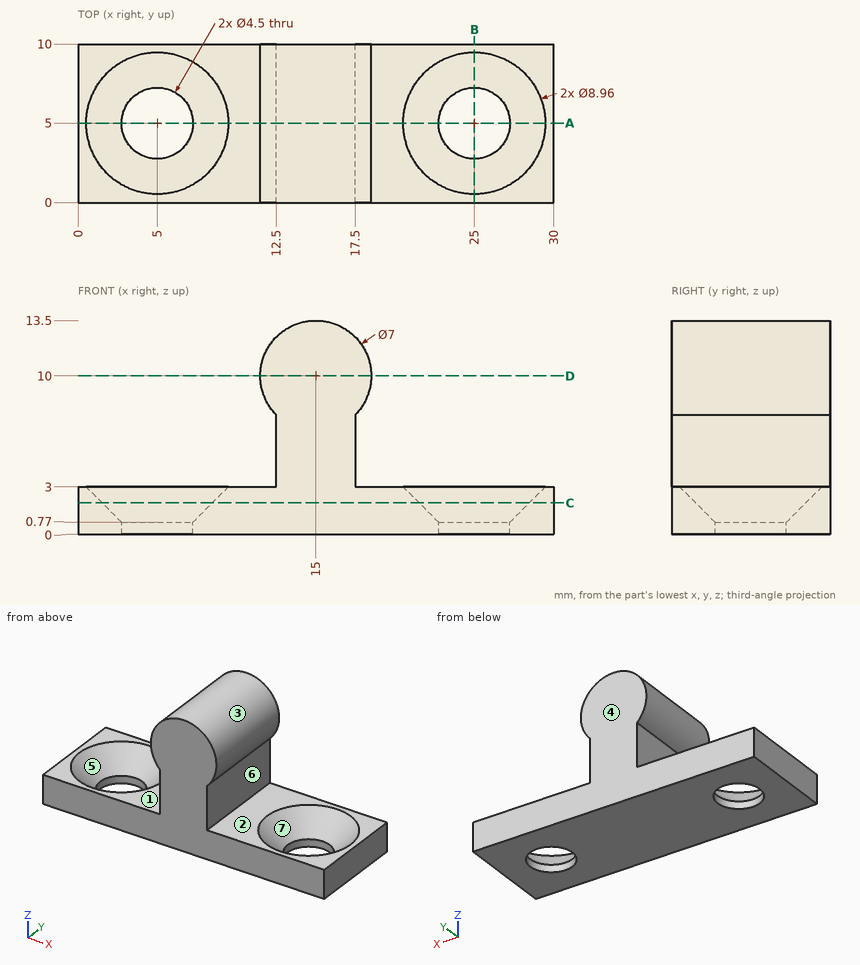
Geometry check sheet. Reference: drawing and pictorial views, mm from the part's lowest x, y, z. A direction names the side the tool comes from. Coordinates: 2 decimals unless noted, no trailing zeros. Order: outer loops, then holes, each group sorted by start corner. A loop starts at its lowest first (then second) coordinate and runs counter-clockwise, first axis right, second up.
Item 1: Scan lines: line 1 along X through (y, z) = (5, 0.4); line 2 along Y through (x, z) = (25, 0.4); line 3 along X through (y, z) = (5, 2.5). Record each from-to range of solid material in increasing order.
Item 2: Depth check by flat-ended pin: pin 1 (4 mm diameter, centred on x = 25, y = 5, fed in from -Z); pin 2 (6 mm diameter, centred on x = 5, y = 5, fed in from +Z); pin 3 (5 mm diameter, centred on y = 5, z = 6, fed in from -X); pin 4 (4 mm diameter, centred on y = 5.5, z = 6.5, fed in from +X). Enter the tip coordinate at first touch or a pass-through.
Item 3: Section check C-C (z = 2). Enter the section's corners in (x, y).
Item 4: Section check D-D (z = 10). Enter the section's corners in (x, y).
Item 5: Section check A-A (y = 5). Enter the section's corners in (x, z).
Item 6: Section check B-B (x = 25). Enter the section's corners in (y, z).
Item 7: Mould release check, pull along X, two halves, no side actions. Record for the marked faces 4, 5, 6 and 7: released by +X, released by -X, zero draft, split by the parting line, or undercut.
Item 8: Tool access check on the marked faces 1, 2 and 3. Record the directions out of +Z, -Z, +X, -X, +Y, -Y that give a thin tool (end or side, any length) a straight path to the whole face; none if there is none.
Check sheet entries:
1. line 1: x = 0 to 2.75, 7.25 to 22.75, 27.25 to 30
1. line 2: y = 0 to 2.75, 7.25 to 10
1. line 3: x = 0 to 1.02, 8.98 to 21.02, 28.98 to 30
2. pin 1: passes through
2. pin 2: stops at z = 1.52
2. pin 3: stops at x = 11.84
2. pin 4: stops at x = 18.16
3. outline: (0, 0) - (30, 0) - (30, 10) - (0, 10) - close; hole circle Ø6.96 at (5, 5); hole circle Ø6.96 at (25, 5)
4. outline: (11.5, 0) - (18.5, 0) - (18.5, 10) - (11.5, 10) - close
5. outline: (0, 0) - (2.75, 0) - (2.75, 0.77) - (0.52, 3) - (0, 3) - close; (7.25, 0) - (22.75, 0) - (22.75, 0.77) - (20.52, 3) - (17.5, 3) - (17.5, 7.55) arc R3.5 ccw (long way) to (12.5, 7.55) - (12.5, 3) - (9.48, 3) - (7.25, 0.77) - close; (27.25, 0) - (30, 0) - (30, 3) - (29.48, 3) - (27.25, 0.77) - close
6. outline: (0, 0) - (2.75, 0) - (2.75, 0.77) - (0.52, 3) - (0, 3) - close; (7.25, 0) - (10, 0) - (10, 3) - (9.48, 3) - (7.25, 0.77) - close
7. face 4: zero draft
7. face 5: undercut
7. face 6: released by +X
7. face 7: undercut
8. face 1: -X, +Y, -Y
8. face 2: +X, +Y, -Y
8. face 3: +Y, -Y
